The listing builds one solid part. Answer for the finished solid, in the listing's coordinates (mm). A direction names the side the tool comes from. Round coordinates to 2 decimals unless told otherwise and drop trailing zeros. Write each loop counter-clockwise with the first axis right and the second up, starting at its lowest first coordinate (ties: lowest second). Pieces come first, ordered by that corner, then holes.
from build123d import *

# Parameters (mm, degrees)
SKETCH1_W           = 20.5
SKETCH1_H           = 5
BOSS_EXTRUDE1_DEPTH = 30


with BuildPart() as part:
    # Sketch1 → Boss-Extrude1 (new body)
    with BuildSketch(Plane.XY):
        with BuildLine():
            Line((17, -18.493179267), (10.25, -18.493179267))
            Line((10.25, -18.493179267), (10.25, -68))
            ThreePointArc((10.25, -68), (0, -78.25), (-10.25, -68))
            Line((-10.25, -68), (-10.25, -18.493179267))
            Line((-10.25, -18.493179267), (-17, -18.493179267))
            Line((-17, -18.493179267), (-17, -68))
            ThreePointArc((-17, -68), (0, -85), (17, -68))
            Line((17, -68), (17, -18.493179267))
        make_face()
        with BuildLine():
            Line((10.25, -68), (10.25, -18.493179267))
            Line((10.25, -18.493179267), (-10.25, -18.493179267))
            Line((-10.25, -18.493179267), (-10.25, -68))
            ThreePointArc((-10.25, -68), (0, -57.75), (10.25, -68))
        make_face()
        with Locations((0, -15.993179267)):
            Rectangle(SKETCH1_W, SKETCH1_H)
        with BuildLine():
            Line((10.25, -13.493179267), (10.25, 0))
            ThreePointArc((10.25, 0), (0, -10.25), (-10.25, 0))
            Line((-10.25, 0), (-10.25, -13.493179267))
            Line((-10.25, -13.493179267), (10.25, -13.493179267))
        make_face()
        with BuildLine():
            ThreePointArc((-10.25, 0), (0, -10.25), (10.25, 0))
            Line((10.25, 0), (-10.25, 0))
        make_face()
        with BuildLine():
            Line((-10.25, 0), (10.25, 0))
            ThreePointArc((10.25, 0), (0, 10.25), (-10.25, 0))
        make_face()
    extrude(amount=BOSS_EXTRUDE1_DEPTH)


solid = part.part
1. A tool of negligible diameter and unlimited length cuts with its end or side. For faces 5 (the face through (10.25, -9, 15)), 6 (the face through (0, -37, 0)), 7 (the face through (-14, -18.493, 15)), from which of +Z, -Z, +X, -X, +Y, -Y can it reach the whole face along a straight path? Write none if from no direction.
Geometry says:
face 5: +Z, -Z, +X, +Y
face 6: -Z, +X, -X, +Y, -Y
face 7: +Z, -Z, -X, +Y
2. Straight lines are drawn through the part: line 1 along Y through (x, z) = (0, 19.25); line 2 along Y through (x, z) = (-8, 11.75); line 3 along X through (y, z) = (-62.5, 15.25). For each, find the intervals that lie inside material, in ascending order.
Geometry says:
line 1: y = -85 to -78.25, -57.75 to 10.25
line 2: y = -83 to -74.41, -61.59 to 6.41
line 3: x = -17 to -8.65, 8.65 to 17
3. Section C-C on y = -17.5 is taken. Determine the outline of the cut face in (x, z).
Geometry says:
outline: (-10.25, 0) - (10.25, 0) - (10.25, 30) - (-10.25, 30) - close
4. For a pull along X with two mould halves and no side action, classify faces 1 (the face through (-4.73, -77.094, 14.79)), 2 (the face through (14, -18.493, 15)), 3 (the face through (-10.25, -9, 15)), 4 (the face through (17, -44, 15)) as released by +X, released by -X, zero draft, split by the parting line, or undercut.
Geometry says:
face 1: undercut
face 2: zero draft
face 3: released by -X
face 4: released by +X
5. Given pin 1 (3 mm diameter, centred on y = -12.5, z = 16, fed in from +X); pin 2 (2 mm diameter, centred on x = 12.5, z = 13.5, fed in from +Y); pin 3 (16.5 mm diameter, centred on x = 0, y = -68, fed in from +Z); pin 4 (5 mm diameter, centred on x = 4.5, z = 27, fed in from +Y), each flat-ended and moving along its own axis, determine where each tip first touches the part or whether it passes through.
Geometry says:
pin 1: stops at x = 10.25
pin 2: stops at y = -18.49
pin 3: passes through
pin 4: stops at y = 10.05
6. Section A-A on x = 0 is taken. Determine the outline of the cut face in (y, z).
Geometry says:
outline: (-85, 0) - (-78.25, 0) - (-78.25, 30) - (-85, 30) - close; (-57.75, 0) - (10.25, 0) - (10.25, 30) - (-57.75, 30) - close
7. Section B-B on z = 20.75 is taken. Determine the outline of the cut face in (x, y).
Geometry says:
outline: (-17, -68) arc R17 ccw to (17, -68) - (17, -18.49) - (10.25, -18.49) - (10.25, 0) arc R10.25 ccw to (-10.25, 0) - (-10.25, -18.49) - (-17, -18.49) - close; hole circle Ø20.5 at (0, -68)
8. Section D-D on x = 8 is taken. Determine the outline of the cut face in (y, z), plus the area to 3 significant figures.
Geometry says:
outline: (-83, 0) - (-74.41, 0) - (-74.41, 30) - (-83, 30) - close; (-61.59, 0) - (6.41, 0) - (6.41, 30) - (-61.59, 30) - close
area: 2,300 mm2
